```python
from build123d import *

# Parameters (mm, degrees)
BOSS_EXTRU_1_DEPTH                                = 20
CHAMBRAGE_POUR_VIS_SIX_PANS_CREUX_M41_D           = 4.5
CHAMBRAGE_POUR_VIS_SIX_PANS_CREUX_M41_DEPTH       = 11.55
CHAMBRAGE_POUR_VIS_SIX_PANS_CREUX_M41_CBORE_D     = 8
CHAMBRAGE_POUR_VIS_SIX_PANS_CREUX_M41_CBORE_DEPTH = 1
ESQUISSE6_W                                       = 20.2
ESQUISSE6_H                                       = 40
ENL_V_MAT_EXTRU_1_DEPTH                           = 3
ESQUISSE16_R                                      = 101.2
ESQUISSE16_R_2                                    = 100
EXTRU_MINCE1_DEPTH                                = 45
ESQUISSE14_W                                      = 30.8
ESQUISSE14_H                                      = 45
BOSS_EXTRU_3_DEPTH                                = 40


with BuildPart() as part:
    # Base → Boss.-Extru.1 (new, symmetric)
    with BuildSketch(Plane(origin=(0, 0, 0), x_dir=(1, 0, 0), z_dir=(0, 1, 0))):
        Polygon((-3.85, -2.4), (-3.85, 2.4), (-10.1, 2.4), (-10.1, 10.1), (-2.4, 10.1), (-2.4, 3.85), (2.4, 3.85), (2.4, 10.1), (10.1, 10.1), (10.1, 2.4), (3.85, 2.4), (3.85, -2.4), (10.1, -2.4), (10.1, -6.25), (15.4, -6.25), (15.4, 15.4), (-15.4, 15.4), (-15.4, -6.25), (-10.1, -6.25), (-10.1, -2.4), align=None)
    extrude(amount=BOSS_EXTRU_1_DEPTH, both=True)

    # Chambrage pour vis à six pans creux M41
    with Locations(Plane(origin=(15.4, 0, 0), x_dir=(0, 0, -1), z_dir=(1, 0, 0))):
        with Locations((0, 0)):
            chambrage_pour_vis_six_pans_creux_m41 = CounterBoreHole(CHAMBRAGE_POUR_VIS_SIX_PANS_CREUX_M41_D / 2, CHAMBRAGE_POUR_VIS_SIX_PANS_CREUX_M41_CBORE_D / 2, CHAMBRAGE_POUR_VIS_SIX_PANS_CREUX_M41_CBORE_DEPTH, depth=CHAMBRAGE_POUR_VIS_SIX_PANS_CREUX_M41_DEPTH)

    # Symétrie1: Chambrage pour vis à six pans creux M41 across plane
    add(chambrage_pour_vis_six_pans_creux_m41.mirror(Plane(origin=(0, 0, 0), x_dir=(0, 0, 1), z_dir=(1, 0, 0))), mode=Mode.SUBTRACT)

    # Esquisse6 → Enlèv. mat.-Extru.1 (cut, symmetric)
    with BuildSketch(Plane.XY):
        Rectangle(ESQUISSE6_W, ESQUISSE6_H)
    extrude(amount=ENL_V_MAT_EXTRU_1_DEPTH, both=True, mode=Mode.SUBTRACT)

    # Esquisse16 → Extru.-Mince1 (add)
    with BuildSketch(Plane(origin=(0, 0, -15.4), x_dir=(-1, 0, 0), z_dir=(0, 0, -1))):
        with Locations((0, -117.566500624)):
            Circle(ESQUISSE16_R)
        with Locations((0, -117.566500624)):
            Circle(ESQUISSE16_R_2, mode=Mode.SUBTRACT)
    extrude(amount=EXTRU_MINCE1_DEPTH)

    # Esquisse14 → Boss.-Extru.3 (add)
    with BuildSketch(Plane.XZ.offset(20)):
        with Locations((0, -37.9)):
            Rectangle(ESQUISSE14_W, ESQUISSE14_H)
    extrude(amount=-BOSS_EXTRU_3_DEPTH)


solid = part.part
```
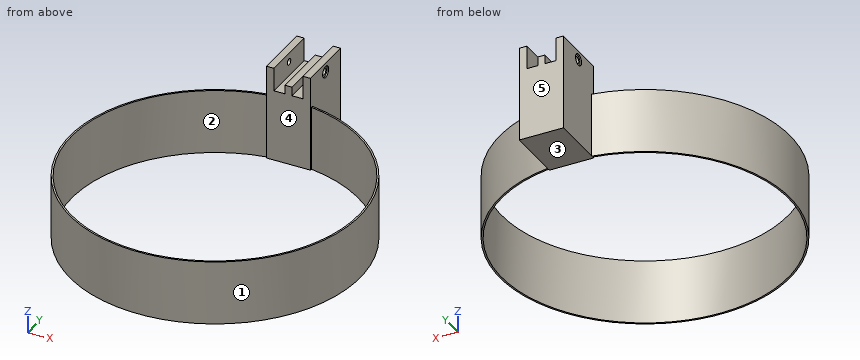
Check sheet for the modelled part. Datum: model origin and axes. Units: mm. Face numbers are marked on the shaded views. A direction names the side the tool comes from. Give positions to 0.01 mm unless a question says otherwise; leave off trailing zeros. Loops run counter-clockwise (first coordinate to the right, second up) from the corner with the lowest first, then second, coordinate; pieces in that order, holes last. Notation, with made-up numbers: (46.25, 5) - (85.25, 5) arc R29 cw to (85.25, 28) - close; hole circle Ø10 at (54, 68.25). An arc over 180 degrees is marked (long way). One line per question, with ' | ' between items. Start each with the question number.
1. Gauge pin test, flat ends, axial feed: pin 1 Ø4 at (y, z) = (-0.5, -2) entering from +X; pin 2 Ø12 at (x, y) = (60, -33) entering from +Z; pin 3 Ø4 at (x, z) = (45.5, -25) entering from +Y. Record the tip position at first contact, or that the pin passes through.
2. Material ranges on line 1 along Y through (x, z) = (-11, 0); line 2 along Y through (x, z) = (14.8, 0); line 3 along X through (y, z) = (-94, -21.5), recorded low to high. Write a range as [from, to].
3. Set-up check for the marked faces 4 and 5: record each of +Z, -Z, +X, -X, +Y, -Y from which the full face is reachable in a straight line by a thin tool's end or side.
4. Draft check along X on the marked faces 1, 2 and 3. Enter one of: released by +X, released by -X, zero draft, split by the parting line, or undercut.
5. Cross-section at A-A, the plane y = -84. Enter the section's corners in (x, z).
6. Cross-section at B-B, the plane x = -53. Enter the section's corners in (y, z).
Check result:
1) pin 1: stops at x = 15.4 | pin 2: stops at z = -15.4 | pin 3: stops at y = -26.19
2) line 1: y = [-20, -2.25], [2.25, 20] | line 2: y = [-20, -4], [4, 20] | line 3: x = [-98.42, -97.18], [97.18, 98.42]
3) face 4: +Z, -Z | face 5: +Z, -Z, +X, -X, +Y
4) face 1: split by the parting line | face 2: undercut | face 3: zero draft
5) outline: (-95.47, -60.4) - (-94.2, -60.4) - (-94.2, -15.4) - (-95.47, -15.4) - close; (94.2, -60.4) - (95.47, -60.4) - (95.47, -15.4) - (94.2, -15.4) - close
6) outline: (-203.78, -60.4) - (-202.37, -60.4) - (-202.37, -15.4) - (-203.78, -15.4) - close; (-32.77, -60.4) - (-31.35, -60.4) - (-31.35, -15.4) - (-32.77, -15.4) - close
